For this review, use the dimensioned drawing (mm, ordinates from the lowest corner) and the shaded views. Round coordinates to 2 decimals unless told otherwise and drop trailing zeros. Order: outer loops, then holes, each group sorted by start corner. A loop starts at its lowest first (then second) coordinate and runs counter-clockwise, first axis right, second up. Notation, with made-up numbers: (21.5, 46) -> (47.5, 46) arc R22 ccw to (47.5, 64) -> close; hole circle Ø1 at (27, 81.5). An arc over 180 degrees is marked (long way). Use a Markdown table: item, result. Add a question column.
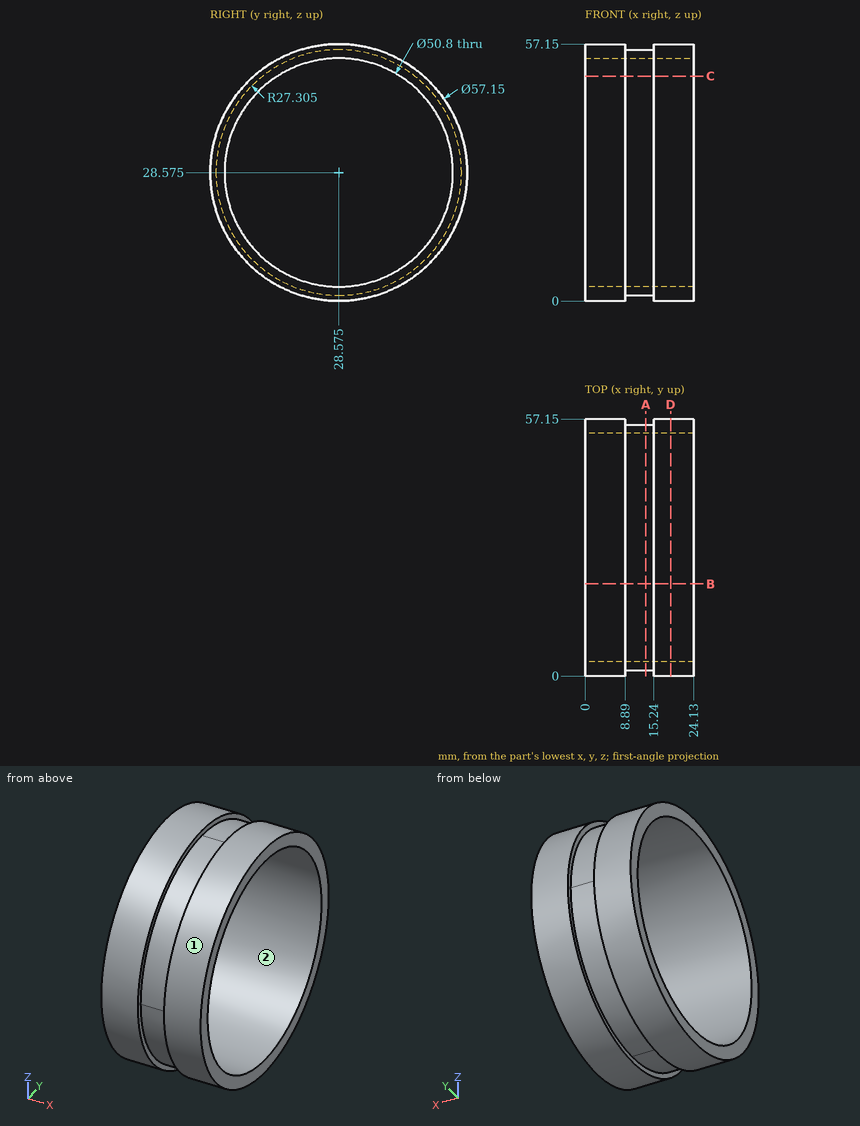
Q1. Wall thickness on line 1 (Y direction, x = 9.75, z = 14); line 2 (Z direction, x = 11.5, y = 50); line 3 (Z direction, x = 5, y = 9): over which ranges is each line inside the solid? List them lowest first. Write a range as [from, to].
Q2. Add section C-C (z = 50). Write out the cut boundary in (x, y).
Q3. Insertion check: pin 1 (5 mm diameter, centred on x = 3, y = 21.5, fed in from +Z); pin 2 (3 mm diameter, centred on x = 6, z = 37, fed in from +Y); pin 3 (4 mm diameter, centred on x = 18, y = 15.5, fed in from +Z); pin 4 (8 mm diameter, centred on y = 10.5, z = 42, fed in from -X). Each pin has a flat end and moves straight along its axis. Give the tip position at first contact, or say it passes through.
Q4. Add section D-D (x = 19). Write out the cut boundary in (y, z) (3 decimals).
Q5. Add section B-B (y = 20.5). Write out the cut boundary in (x, z), then the cut area to 3 significant figures.
Q6. Mouldability with a two-part tool opening along Y and no side actions: class the marked faces 1 and 2 as pulls with the +Y half, pulls with the -Y half, needs draft (parallel to the pull), parting line crosses it, or undercut.
Q7. Add section A-A (x = 13.5). Write out the cut boundary in (y, z) (3 decimals), then the cut area to 3 significant figures.
Report:
| question | item | result |
|---|---|---|
| 1 | line 1 | y = [5.49, 7.77], [49.38, 51.66] |
| 1 | line 2 | z = [11.65, 14.93], [42.22, 45.5] |
| 1 | line 3 | z = [7.76, 12.39], [44.76, 49.39] |
| 2 | outline | (0, 9.67) -> (8.89, 9.67) -> (8.89, 11.65) -> (15.24, 11.65) -> (15.24, 9.67) -> (24.13, 9.67) -> (24.13, 14.93) -> (0, 14.93) -> close; (0, 42.22) -> (24.13, 42.22) -> (24.13, 47.48) -> (15.24, 47.48) -> (15.24, 45.5) -> (8.89, 45.5) -> (8.89, 47.48) -> (0, 47.48) -> close |
| 3 | pin 1 | stops at z = 56.78 |
| 3 | pin 2 | stops at y = 56.3 |
| 3 | pin 3 | stops at z = 54.92 |
| 3 | pin 4 | stops at x = 0 |
| 4 | outline | circle Ø57.15 at (28.575, 28.575); hole circle Ø50.8 at (28.575, 28.575) |
| 5 | outline | (0, 1.16) -> (8.89, 1.16) -> (8.89, 2.49) -> (15.24, 2.49) -> (15.24, 1.16) -> (24.13, 1.16) -> (24.13, 4.49) -> (0, 4.49) -> close; (0, 52.66) -> (24.13, 52.66) -> (24.13, 55.99) -> (15.24, 55.99) -> (15.24, 54.66) -> (8.89, 54.66) -> (8.89, 55.99) -> (0, 55.99) -> close |
| 5 | area | 144 mm² |
| 6 | face 1 | parting line crosses it |
| 6 | face 2 | undercut |
| 7 | outline | circle Ø54.61 at (28.575, 28.575); hole circle Ø50.8 at (28.575, 28.575) |
| 7 | area | 315 mm² |
